Autodesk Inventor part; units mm, degrees
ref_plane "YZ Plane" through (0, 0, 0) normal (1, 0, 0) x (0, 1, 0)
ref_plane "XZ Plane" through (0, 0, 0) normal (0, 1, 0) x (-1, 0, 0)
ref_plane "XY Plane" through (0, 0, 0) normal (0, 0, 1) x (1, 0, 0)
ref_plane "Work Plane1" through (0, 0, 0) normal (0, 0, 1) x (1, 0, 0)
sketch "Sketch1" plane through (0, 0, 0) normal (0, 0, 1) x (1, 0, 0)
  circle A0 centre (15.5, -15.5) radius 1.7
  circle A1 centre (15.5, 15.5) radius 1.7
  circle A2 centre (-15.5, 15.5) radius 1.7
  circle A3 centre (-15.5, -15.5) radius 1.7
  circle A4 centre (0, 0) radius 11
  line L0 (17.5, 21) -> (21, 17.5)
  line L1 (17.5, 21) -> (-17.5, 21)
  line L2 (-21, 17.5) -> (-17.5, 21)
  line L3 (-21, 17.5) -> (-21, -17.5)
  line L4 (-17.5, -21) -> (-21, -17.5)
  line L5 (-17.5, -21) -> (17.5, -21)
  line L6 (21, -17.5) -> (17.5, -21)
  line L7 (21, -17.5) -> (21, 17.5)
  line L8 (-31, 21) -> (239, 21)
  line L9 (239, 21) -> (239, -66)
  line L10 (239, -66) -> (-31, -66)
  line L11 (-31, -66) -> (-31, 21)
  circle A5 centre (207, 0) radius 22 construction
  line L12 (0, 0) -> (239, 0) construction
  circle A6 centre (0, 0) radius 11.5
  line L13 (104, 21) -> (104, -66) construction
  line L14 (-15.5, 15.5) -> (-31, 15.5) construction
  line L15 (207, 0) -> (207, -66) construction
  line L16 (0, 0) -> (0, -66) construction
  line L17 (219.5, -49) -> (194.5, -49)
  line L18 (194.5, -49) -> (194.5, -61)
  line L19 (194.5, -61) -> (219.5, -61)
  line L20 (219.5, -61) -> (219.5, -49)
  line L21 (219.5, -49) -> (194.5, -61) construction
  line L22 (194.5, -49) -> (219.5, -61) construction
  line L23 (219.5, -55) -> (194.5, -55) construction
  line L24 (-13.5, -61) -> (13.5, -61)
  line L25 (13.5, -61) -> (13.5, -49)
  line L26 (13.5, -49) -> (-13.5, -49)
  line L27 (-13.5, -49) -> (-13.5, -61)
  line L28 (-13.5, -61) -> (13.5, -49) construction
  line L29 (13.5, -61) -> (-13.5, -49) construction
  line L30 (170, 23) -> (166.5, 26.5)
  line L31 (170, 23) -> (170, -12)
  line L32 (166.5, -15.5) -> (170, -12)
  line L33 (166.5, -15.5) -> (131.5, -15.5)
  line L34 (128, -12) -> (131.5, -15.5)
  line L35 (128, -12) -> (128, 23)
  line L36 (131.5, 26.5) -> (128, 23)
  line L37 (131.5, 26.5) -> (166.5, 26.5)
  line L38 (127.5, 23.2071) -> (127.5, -12.2071)
  line L39 (127.5, -12.2071) -> (131.2929, -16)
  line L40 (131.2929, -16) -> (166.7071, -16)
  line L41 (166.7071, -16) -> (170.5, -12.2071)
  line L42 (170.5, -12.2071) -> (170.5, 23.2071)
  line L43 (170.5, 23.2071) -> (166.7071, 27)
  line L44 (166.7071, 27) -> (131.2929, 27)
  line L45 (131.2929, 27) -> (127.5, 23.2071)
  line L46 (-32.0916, -17) -> (139.8961, -17) construction
  point P0 (-26, 15.5)
  point P1 (-26, -14)
  point P2 (234, 15.5)
  point P3 (234, -14)
  point P4 (207, -55)
  point P5 (226.5, -55)
  point P6 (187.5, -55)
  point P7 (0, -55)
  point P8 (20.5, -55)
  point P9 (-18.5, -55)
  point P10 (26, 15.5)
  point P11 (26, -14)
  point P12 (180, 15.5)
  point P13 (180, -14)
  point P14 (170.5, 21)
  point P15 (127.5, 21)
  dimension "d0" = 45
  dimension "d1" = 270
  dimension "d2" = 44
  dimension "d3" = 0.5
  dimension "d21" = 10
  dimension "d22" = 32
  dimension "d23" = 5
  dimension "d31" = 25
  dimension "d32" = 12
  dimension "d33" = 5
  dimension "d34" = 7
  dimension "d42" = 0.5
  dimension "d50" = 5
  dimension "d51" = 17
  dimension "d52" = 3
extrude "Extrusion1" add sketch "Sketch1" along normal blind 4 contours A0 | A1 | A2 | A3 | A4 | L8 L38 L39 L40 L41 L42 L9 L10 L11 L2 L3 L4 L5 L6 L7 L0 | L0 L7 L6 L5 L4 L3 L2 L1 | A6
hole "Hole1" at (207, 0, 0) direction (0, 0, 1) diameter 5.5 end through all
sketch "Sketch2" plane through (0, 0, 4) normal (0, 0, 1) x (1, 0, 0)
  circle A0 centre (15.5, -15.5) radius 1.7
  circle A1 centre (15.5, 15.5) radius 1.7
  circle A2 centre (-15.5, 15.5) radius 1.7
  circle A3 centre (-15.5, -15.5) radius 1.7
  circle A4 centre (0, 0) radius 11
  line L0 (17.5, 21) -> (21, 17.5)
  line L1 (17.5, 21) -> (-17.5, 21)
  line L2 (-21, 17.5) -> (-17.5, 21)
  line L3 (-21, 17.5) -> (-21, -17.5)
  line L4 (-17.5, -21) -> (-21, -17.5)
  line L5 (-17.5, -21) -> (17.5, -21)
  line L6 (21, -17.5) -> (17.5, -21)
  line L7 (21, -17.5) -> (21, 17.5)
  point P0 (-18.5, -55)
  point P1 (20.5, -55)
  point P2 (187.5, -55)
  point P3 (226.5, -55)
fillet "Fillet1" radius 5 4 edges at (-31, 21, 2) (-31, -66, 2) (239, 21, 2) (239, -66, 2)
hole "Hole3" at (-26, -14, 0) at (-26, 15.5, 0) at (234, 15.5, 0) at (234, -14, 0) at (26, 15.5, 0) at (26, -14, 0) direction (0, 0, 1) diameter 3.4 end through all countersink diameter 6.6 countersink angle 90
hole "Hole4" at (-18.5, -55, 4) at (20.5, -55, 4) at (187.5, -55, 4) at (226.5, -55, 4) direction (0, 0, -1) diameter 3.4 end through all countersink diameter 6.6 countersink angle 90
hole "Hole5" at (180, 15.5, 0) at (180, -14, 0) direction (0, 0, 1) diameter 3.4 end through all
hole "Hole6" at (0, 0, 0) direction (0, 0, 1) diameter 5.5 depth 8
properties part number "plate_1"
The listing builds one solid part. Answer for the finished solid, in the listing's coordinates (mm). Coordinates: 2 decimals unless noted, no trailing zeros. Order: outer loops, then holes, each group sorted by start corner. A loop starts at its lowest first (then second) coordinate and runs counter-clockwise, first axis right, second up. Notation, with made-up numbers: (3, 26.25) -> (19, 26.25) arc R30 ccw to (19, 48.25) -> close; hole circle Ø7 at (79.25, 34). An arc over 180 degrees is marked (long way). Answer in a Markdown table with one row per item. Add a question column.
Item 1: Find section A-A (x = 0). Write down the section's boundary in (y, z).
Item 2: Each of these flat-tipped pins is pushed along its axis until it touches: P1, Ø4, axis at x = 26, y = -14, coming from the -Z side; P2, Ø5.5, axis at x = 187.5, y = -55, coming from the +Z side; P3, Ø2, axis at x = 154, z = 2, coming from the +Y side. Where does it stop, or does it pass through?
Item 3: Determine the mould class of faces 1 (the face through (209.685, -0.596, 2.028)), 2 (the face through (-29, 20, 2)), 3 (the face through (237, -65, 2)) for opening direction Y: +Y half, -Y half, draft (parallel to the pull), parting line (faces both ways), or undercut.
Item 4: Find the intervals of material crossed by L1, parallel to Y at x = 0, z = 2.1; L2, parallel to Y at x = -26, z = 2.95; L3, parallel to X at y = 15.5, z = 3.45, in increasing order. Write a range as from..to.
Item 5: Find section C-C (x = 154.5). Write down the section's boundary in (y, z), then the cut area to 3 significant figures.
Item 6: Find section B-B (z = 3.25). State how many separate pieces and enclosed holes the cut face has, then the cut area to 3 significant figures.
Result set:
| question | item | result |
|---|---|---|
| 1 | outline | (-66, 0) -> (-61, 0) -> (-61, 4) -> (-66, 4) -> close; (-49, 0) -> (-2.75, 0) -> (-2.75, 4) -> (-49, 4) -> close; (2.75, 0) -> (21, 0) -> (21, 4) -> (2.75, 4) -> close |
| 2 | P1 | stops at z = 1.3 |
| 2 | P2 | stops at z = 3.45 |
| 2 | P3 | stops at y = -16 |
| 3 | face 1 | undercut |
| 3 | face 2 | +Y half |
| 3 | face 3 | -Y half |
| 4 | L1 | y = -66..-61, -49..-2.75, 2.75..21 |
| 4 | L2 | y = -66..-15.7, -12.3..13.8, 17.2..21 |
| 4 | L3 | x = -31..-27.7, -24.3..24.3, 27.7..127.5, 170.5..178.3, 181.7..232.3, 235.7..239 |
| 5 | outline | (-66, 0) -> (-16, 0) -> (-16, 4) -> (-66, 4) -> close |
| 5 | area | 200 mm² |
| 6 | separate pieces | 1 |
| 6 | enclosed holes | 16 |
| 6 | area | 21,100 mm² |
